Verification items for this drawing (mm, ordinates from the low corner). A direction names the side the tool comes from. Give positions to 0.01 mm unless a question says otherwise; leave off trailing zeros. Order: outer loops, then holes, each group sorted by start corner. A loop starts at its lowest first (then second) coordinate and runs counter-clockwise, first axis right, second up. Notation, with made-up numbers: M -9.5,14 L 38.5,14 A22 cw 38.5,47 Z; hole C 42.5,-25.5 d7. An arc over 180 degrees is marked long. One line per question, with ' | ' between items. Start each with the question number.
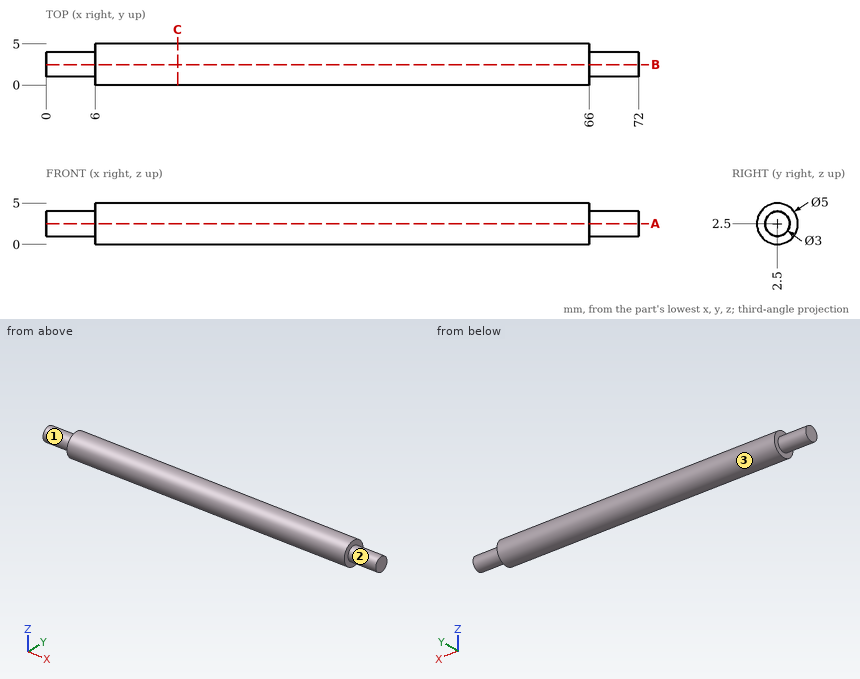
Item 1: Depth check by flat-ended pin: pin 1 (1.5 mm diameter, centred on x = 46, y = 4, fed in from +Z). Enter the tip coordinate at first touch or a pass-through.
Item 2: Cross-section at A-A, the plane z = 2.5. Record the cut outline in (x, y), plus the area to 3 significant figures.
Item 3: Material ranges on line 1 along X through (y, z) = (0.6, 2.1); line 2 along Z through (x, y) = (36.5, 2.7), recorded low to high.
Item 4: Cross-section at C-C, the plane x = 16. Record the cut outline in (y, z).
Item 5: Set-up check for the marked faces 1, 2 and 3: record each of +Z, -Z, +X, -X, +Y, -Y from which the full face is reachable in a straight line by a thin tool's end or side.
Outcome:
1) pin 1: stops at z = 4.88
2) outline: M 0,1 L 6,1 L 6,0 L 66,0 L 66,1 L 72,1 L 72,4 L 66,4 L 66,5 L 6,5 L 6,4 L 0,4 Z | area: 336 mm²
3) line 1: x = 6 to 66 | line 2: z = 0.01 to 4.99
4) outline: C 2.5,2.5 d5
5) face 1: -X | face 2: +X | face 3: +X, -X
